Input: part model. Units: mm. Frame: model coordinates. Round coordinates to 2 decimals unless told otherwise and drop trailing zeros. Loops run counter-clockwise (first coordinate to the right, second up) from the corner with the lowest first, then second, coordinate; pieces in that order, holes last. Notation, with made-up numbers: (17.5, -25) -> (33.5, -25) arc R25 ccw to (33.5, 11) -> close; hole circle Ø5 at (75.5, 39.25). An arc over 180 degrees is marked (long way). Answer as a JSON object with one key per item and string values. Group by question number.
Item 1: Pin query (flat end, axial travel): pin 1 (8 mm diameter, centred on x = -9.5, z = -57, fed in from -Y); pin 2 (1.9 mm diameter, centred on y = 2, z = 49, fed in from -X). Return the tip coordinate at first contact, or that it passes through.
Item 2: Material intervals for line 1 (Z direction, x = -59, y = 1.25); line 2 (Z direction, x = -84, y = 4); line 3 (X direction, y = 3, z = -87), sorted ascending. Write a range as [from, to].
Item 3: Section query B-B on x = 97.5. Return loops of the section in (y, z), and give its area (3 significant figures).
Item 4: Section query D-D on z = 31. Return loops of the section in (x, y).
Item 5: Section query A-A on x = -58.5. Return loops of the section in (y, z).
Item 6: Section query C-C on y = 4.75. Count the separate pieces of the cut face and the enclosed holes in it, and give its area (3 significant figures).
from build123d import *

# Parameters (mm, degrees)
SKETCH1_W           = 304
SKETCH1_H           = 609
BOSS_EXTRUDE1_DEPTH = 6.35
CUT_EXTRUDE1_DEPTH  = 386.382582119
CUT_EXTRUDE3_DEPTH  = 386.382582119


with BuildPart() as part:
    # Sketch1 → Boss-Extrude1 (new body)
    with BuildSketch(Plane(origin=(0, 0, 0), x_dir=(1, 0, 0), z_dir=(0, 1, 0))):
        with Locations((12.142011834, 44.121301775)):
            Rectangle(SKETCH1_W, SKETCH1_H)
    extrude(amount=BOSS_EXTRUDE1_DEPTH)

    # Sketch3 → Cut-Extrude1 (cut, through all)
    with BuildSketch(Plane(origin=(0, 6.35, 0), x_dir=(1, 0, 0), z_dir=(0, 1, 0))):
        with BuildLine():
            Line((154.142011834, -120.378698225), (54.142011834, -120.378698225))
            ThreePointArc((54.142011834, -120.378698225), (47.070944022, -117.449766037), (44.142011834, -110.378698225))
            Line((44.142011834, -110.378698225), (44.142011834, -10.378698225))
            ThreePointArc((44.142011834, -10.378698225), (47.070944022, -3.307630413), (54.142011834, -0.378698225))
            Line((54.142011834, -0.378698225), (154.142011834, -0.378698225))
            ThreePointArc((154.142011834, -0.378698225), (161.213079646, -3.307630413), (164.142011834, -10.378698225))
            Line((164.142011834, -10.378698225), (164.142011834, -110.378698225))
            ThreePointArc((164.142011834, -110.378698225), (161.213079646, -117.449766037), (154.142011834, -120.378698225))
        make_face()
        with BuildLine():
            Line((-129.857988166, -120.378698225), (-29.857988166, -120.378698225))
            ThreePointArc((-29.857988166, -120.378698225), (-22.786920354, -117.449766037), (-19.857988166, -110.378698225))
            Line((-19.857988166, -110.378698225), (-19.857988166, -10.378698225))
            ThreePointArc((-19.857988166, -10.378698225), (-22.786920354, -3.307630413), (-29.857988166, -0.378698225))
            Line((-29.857988166, -0.378698225), (-129.857988166, -0.378698225))
            ThreePointArc((-129.857988166, -0.378698225), (-136.929055978, -3.307630413), (-139.857988166, -10.378698225))
            Line((-139.857988166, -10.378698225), (-139.857988166, -110.378698225))
            ThreePointArc((-139.857988166, -110.378698225), (-136.929055978, -117.449766037), (-129.857988166, -120.378698225))
        make_face()
    extrude(amount=-CUT_EXTRUDE1_DEPTH, mode=Mode.SUBTRACT)

    # Sketch4 → Cut-Extrude3 (cut, through all)
    with BuildSketch(Plane(origin=(0, 6.35, 0), x_dir=(1, 0, 0), z_dir=(0, 1, 0))):
        with BuildLine():
            Line((20.906944625, 141.682393226), (76.906944625, 141.682393226))
            ThreePointArc((76.906944625, 141.682393226), (81.856692093, 139.632140694), (83.906944625, 134.682393226))
            Line((83.906944625, 134.682393226), (83.906944625, 78.682393226))
            ThreePointArc((83.906944625, 78.682393226), (81.856692093, 73.732645757), (76.906944625, 71.682393226))
            Line((76.906944625, 71.682393226), (20.906944625, 71.682393226))
            ThreePointArc((20.906944625, 71.682393226), (15.957197157, 73.732645757), (13.906944625, 78.682393226))
            Line((13.906944625, 78.682393226), (13.906944625, 134.682393226))
            ThreePointArc((13.906944625, 134.682393226), (15.957197157, 139.632140694), (20.906944625, 141.682393226))
        make_face()
        with BuildLine():
            Line((-82.776888169, 202.809428977), (-26.776888169, 202.809428977))
            ThreePointArc((-26.776888169, 202.809428977), (-21.8271407, 200.759176445), (-19.776888169, 195.809428977))
            Line((-19.776888169, 195.809428977), (-19.776888169, 139.809428977))
            ThreePointArc((-19.776888169, 139.809428977), (-21.8271407, 134.859681509), (-26.776888169, 132.809428977))
            Line((-26.776888169, 132.809428977), (-82.776888169, 132.809428977))
            ThreePointArc((-82.776888169, 132.809428977), (-87.726635637, 134.859681509), (-89.776888169, 139.809428977))
            Line((-89.776888169, 139.809428977), (-89.776888169, 195.809428977))
            ThreePointArc((-89.776888169, 195.809428977), (-87.726635637, 200.759176445), (-82.776888169, 202.809428977))
        make_face()
    extrude(amount=-CUT_EXTRUDE3_DEPTH, mode=Mode.SUBTRACT)


solid = part.part
Solved:
{
 "1": {"pin 1": "y = 0", "pin 2": "x = -19.86"},
 "2": {"line 1": "[-348.62, -202.81], [-132.81, 0.38], [120.38, 260.38]", "line 2": "[-348.62, -202.7], [-132.92, 0.38], [120.38, 260.38]", "line 3": "[-139.86, 13.91], [83.91, 164.14]"},
 "3": {"outline": "(0, -348.62) -> (6.35, -348.62) -> (6.35, 0.38) -> (0, 0.38) -> close; (0, 120.38) -> (6.35, 120.38) -> (6.35, 260.38) -> (0, 260.38) -> close", "area": "3,110 mm²"},
 "4": {"outline": "(-19.86, 0) -> (44.14, 0) -> (44.14, 6.35) -> (-19.86, 6.35) -> close"},
 "5": {"outline": "(0, -348.62) -> (6.35, -348.62) -> (6.35, -202.81) -> (0, -202.81) -> close; (0, -132.81) -> (6.35, -132.81) -> (6.35, 0.38) -> (0, 0.38) -> close; (0, 120.38) -> (6.35, 120.38) -> (6.35, 260.38) -> (0, 260.38) -> close"},
 "6": {"separate pieces": "1", "enclosed holes": "2", "area": "147,000 mm²"}
}
